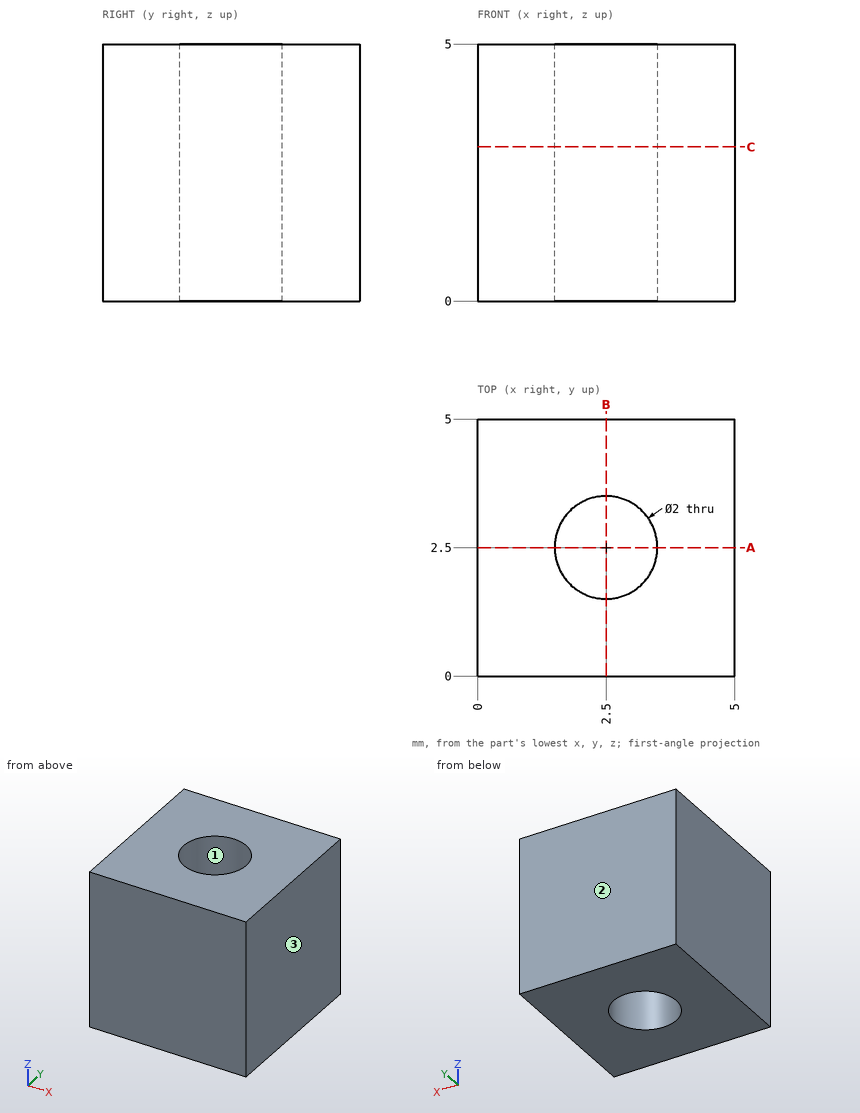
Input: dimensioned drawing with shaded views. Units: mm. Origin: part minimum x, y, z. Give positions to 0.01 mm unless a question says otherwise; leave off trailing zeros. Write each loop counter-clockwise with the first axis right and the second up, starting at its lowest first coordinate (ties: lowest second). Pieces come first, ordered by that corner, then holes.
1. Material intervals for line 1 along Y through (x, z) = (2.5, 1.45); line 2 along X through (y, z) = (2.6, 1.3); line 3 along X through (y, z) = (1.9, 4.05), sorted ascending.
2. Pull-direction query (X, two-part tool) for the marked faces 1, 2 and 3; classes: +X half, -X half, draft (parallel to the pull), parting line (faces both ways), or undercut.
3. Section query A-A (y = 2.5). Return the cut outline in (x, z).
4. Section query C-C (z = 3). Return the cut outline in (x, y).
Output values:
1. line 1: y = 0 to 1.5, 3.5 to 5
1. line 2: x = 0 to 1.51, 3.49 to 5
1. line 3: x = 0 to 1.7, 3.3 to 5
2. face 1: undercut
2. face 2: draft
2. face 3: +X half
3. outline: (0, 0) - (1.5, 0) - (1.5, 5) - (0, 5) - close; (3.5, 0) - (5, 0) - (5, 5) - (3.5, 5) - close
4. outline: (0, 0) - (5, 0) - (5, 5) - (0, 5) - close; hole circle Ø2 at (2.5, 2.5)
